Autodesk Inventor part; units mm, degrees
ref_plane "YZ Plane" through (0, 0, 0) normal (1, 0, 0) x (0, 1, 0)
ref_plane "XZ Plane" through (0, 0, 0) normal (0, 1, 0) x (-1, 0, 0)
ref_plane "XY Plane" through (0, 0, 0) normal (0, 0, 1) x (1, 0, 0)
sketch "Skizze1" plane through (0, 0, 0) normal (0, 0, 1) x (1, 0, 0)
  arc A0 (-370.4, 125) -> (-371.4, 124) centre (-370.4, 124) ccw
  line L0 (-361.6643, 125) -> (-370.4, 125)
  arc A1 (-360.6643, 124) -> (-361.6643, 125) centre (-361.6643, 124) ccw
  line L1 (-360.6643, 120) -> (-360.6643, 124)
  arc A2 (-346.4361, 138.3117) -> (-345.027, 138.6477) centre (-345.8915, 139.1504) ccw
  line L2 (-344.2357, 140.0086) -> (-345.027, 138.6477)
  arc A3 (-344.2357, 140.0086) -> (-344.3931, 141.2184) centre (-345.1002, 140.5113) ccw
  line L3 (-353.1746, 150) -> (-344.3931, 141.2184)
  line L4 (-367.1746, 150) -> (-353.1746, 150)
  line L5 (-375, 128.5) -> (-367.1746, 150)
  line L6 (-375, 120) -> (-375, 128.5)
  line L7 (-371.4, 120) -> (-375, 120)
  line L8 (-371.4, 124) -> (-371.4, 120)
  line L9 (-357.3008, 147) -> (-364.6666, 147) construction
  line L10 (-364.6666, 147) -> (-371.4, 128.5) construction
  line L11 (0, 0) -> (-360, 0) construction
  line L12 (-356.9218, 138.1504) -> (-345, 0) construction
  line L13 (-356.9218, 138.1504) -> (0, 138.1504) construction
  line L14 (0, 138.1504) -> (0, 0) construction
  line L15 (-360, 129.6932) -> (-360, 0) construction
  line L16 (0, 0) -> (-225, 0) construction
  line L17 (-225, 0) -> (-225, 50) construction
  line L18 (-225, 50) -> (0, 50) construction
  line L19 (0, 50) -> (0, 0) construction
  line L20 (-346.4361, 138.3117) -> (-354.8697, 143.7886)
  line L21 (-360, 129.6932) -> (-355.5655, 121.4749)
  arc A4 (-356.4455, 120) -> (-355.5655, 121.4749) centre (-356.4455, 121) ccw
  line L22 (-225, 0) -> (-345, 0) construction
  line L23 (-345, 0) -> (-345, 35) construction
  line L24 (-345, 35) -> (-225, 35) construction
  line L25 (-225, 35) -> (-225, 0) construction
  line L26 (-356.4455, 120) -> (-360.6643, 120)
  line L27 (-354.8697, 143.7886) -> (-360, 129.6932)
  line L28 (-356.9218, 138.1504) -> (0, 8.2415) construction
  line L29 (-363.6, 129.6932) -> (-357.3008, 147) construction
  line L30 (-360, 129.6932) -> (-374.5657, 129.6932) construction
  line L31 (-363.6, 129.6932) -> (-358.3696, 120) construction
  line L32 (-344.2357, 140.0086) -> (-355.581, 120.4973) construction
  arc A5 (-358.9913, 142.3556) -> (-365.4954, 144.7229) centre (-362.2433, 143.5392) ccw
  arc A6 (-369.2753, 134.3376) -> (-362.7712, 131.9703) centre (-366.0232, 133.1539) ccw
  line L33 (-365.4954, 144.7229) -> (-369.2753, 134.3376)
  line L34 (-358.9913, 142.3556) -> (-362.7712, 131.9703)
  line L35 (-371.4, 120) -> (-371.4, 128.5) construction
  dimension "d1" = 30
  dimension "d5" = 1
  dimension "d6" = 1
  dimension "d9" = 135
  dimension "d14" = 8.5
  dimension "d18" = 360
  dimension "d25" = 50
  dimension "d26" = 225
  dimension "d31" = 14
  dimension "d40" = 3.5
  dimension "d41" = 120
  dimension "d42" = 35
  dimension "d43" = 1
  dimension "d47" = 6
  dimension "d50" = 65.068
  dimension "d54" = 15
  dimension "d55" = 3
  dimension "d59" = 12
  dimension "d60" = 160
  dimension "d61" = 120
  dimension "d63" = 3.6
  dimension "d64" = 3.6
  dimension "d65" = 5
  dimension "d66" = 15
revolve "Umdrehung1" add sketch "Skizze1" angle 60 about axis through (0, 138.1504, 0) along (0, -1, 0)
properties part number "LED-Ring_Element"
Source: CAD feature listing. Evaluate the final solid. Frame: model axes, mm. A direction names the side the tool comes from. Round coordinates to 2 decimals unless told otherwise and drop trailing zeros. Use CSV: the item, a comma, the result in double quotes. Start each with the question number.
Q1. First-contact query: P1, Ø1.5, axis at y = 127, z = -195.5, coming from the +X side; P2, Ø5, axis at x = -212, y = 142, coming from the -Z side; P3, Ø10, axis at y = 124, z = -289, coming from the -X side. Flat tips, straight axial feed; report the tip coordinate or a pass-through.
Q2. Line query: line 1 (Z direction, x = -248.5, y = 139.5); line 2 (X direction, y = 143.5, z = -193); line 3 (Y direction, x = -264, z = -244). Output: solid intervals per line, ascending. Write a range as from..to.
Q3. Pull-direction query (X, two-part tool) for faces 4 (the face through (-297.46, 141.77, -174.66)), 5 (the face through (-322, 120, -187)), 6 (the face through (-317, 125, -185)); classes: +X half, -X half, draft (parallel to the pull), parting line (faces both ways), or undercut.
Q4. Access query for faces 1 (the face through (-312.409, 141.706, -177.329)), 2 (the face through (-306.856, 121.989, -180.176)), 3 (the face through (-322.994, 121.972, -183.337)). Directions: +Z, -Z, +X, -X, +Y, -Y. A direction counts if a zero-diameter tool reaches every point of the face in a straight line with its end or side. Return the directions, or none.
Results found:
1,P1,"x = -299.87"
1,P2,"z = -305.4"
1,P3,"x = -244.89"
2,line 1,"-275.47..-270.61, -260.52..-255.52, -244..-238.64"
2,line 2,"-315.14..-310.91, -302.45..-297.92, -297.27..-287.98"
2,line 3,"120..128.75, 131.1..140.99, 145.63..150"
3,face 4,"+X half"
3,face 5,"draft"
3,face 6,"undercut"
4,face 1,"none"
4,face 2,"+Z, +X"
4,face 3,"-Y"
